from build123d import *

# Parameters (mm, degrees)
SALIENTE_EXTRUIR1_DEPTH = 1400
CROQUIS2_R              = 3
CORTAR_EXTRUIR1_DEPTH   = 1401.160705062
CORTAR_EXTRUIR3_DEPTH   = 1401.160705062
CROQUIS4_W              = 1150
CROQUIS4_H              = 72.748415438
CORTAR_EXTRUIR5_DEPTH   = 254


with BuildPart() as part:
    # Croquis1 → Saliente-Extruir1 (new body)
    with BuildSketch(Plane.XY):
        with BuildLine():
            Line((-14, 15), (14, 15))
            ThreePointArc((14, 15), (14.707106781, 14.707106781), (15, 14))
            Line((15, 14), (15, -14))
            ThreePointArc((15, -14), (14.707106781, -14.707106781), (14, -15))
            Line((14, -15), (-14, -15))
            ThreePointArc((-14, -15), (-14.707106781, -14.707106781), (-15, -14))
            Line((-15, -14), (-15, 14))
            ThreePointArc((-15, 14), (-14.707106781, 14.707106781), (-14, 15))
        make_face()
    extrude(amount=-SALIENTE_EXTRUIR1_DEPTH)

    # Croquis2 → Cortar-Extruir1 (cut, through all)
    with BuildSketch(Plane.XY):
        Circle(CROQUIS2_R)
    extrude(amount=-CORTAR_EXTRUIR1_DEPTH, mode=Mode.SUBTRACT)

    # Croquis3 → Cortar-Extruir3 (cut, through all)
    with BuildSketch(Plane.XY):
        with BuildLine():
            Line((-5.492893219, 4.078679656), (-11.292893219, 9.878679656))
            ThreePointArc((-11.292893219, 9.878679656), (-12.382683432, 10.095452408), (-13, 9.171572875))
            Line((-13, 9.171572875), (-13, 5))
            ThreePointArc((-13, 5), (-14, 4), (-15, 5))
            Line((-15, 5), (-15, -5))
            ThreePointArc((-15, -5), (-14, -4), (-13, -5))
            Line((-13, -5), (-13, -9.171572875))
            ThreePointArc((-13, -9.171572875), (-12.382683432, -10.095452408), (-11.292893219, -9.878679656))
            Line((-11.292893219, -9.878679656), (-5.492893219, -4.078679656))
            ThreePointArc((-5.492893219, -4.078679656), (-5.276120467, -3.754256308), (-5.2, -3.371572875))
            Line((-5.2, -3.371572875), (-5.2, 3.371572875))
            ThreePointArc((-5.2, 3.371572875), (-5.276120467, 3.754256308), (-5.492893219, 4.078679656))
        make_face()
        with BuildLine():
            ThreePointArc((-9.171572875, 13), (-10.095452408, 12.382683432), (-9.878679656, 11.292893219))
            Line((-9.878679656, 11.292893219), (-4.078679656, 5.492893219))
            ThreePointArc((-4.078679656, 5.492893219), (-3.754256308, 5.276120467), (-3.371572875, 5.2))
            Line((-3.371572875, 5.2), (3.371572875, 5.2))
            ThreePointArc((3.371572875, 5.2), (3.754256308, 5.276120467), (4.078679656, 5.492893219))
            Line((4.078679656, 5.492893219), (9.878679656, 11.292893219))
            ThreePointArc((9.878679656, 11.292893219), (10.095452408, 12.382683432), (9.171572875, 13))
            Line((9.171572875, 13), (5, 13))
            ThreePointArc((5, 13), (4, 14), (5, 15))
            Line((5, 15), (-5, 15))
            ThreePointArc((-5, 15), (-4.292893219, 14.707106781), (-4, 14))
            ThreePointArc((-4, 14), (-4.292893219, 13.292893219), (-5, 13))
            Line((-5, 13), (-9.171572875, 13))
        make_face()
        with BuildLine():
            Line((9.878679656, -11.292893219), (4.078679656, -5.492893219))
            ThreePointArc((4.078679656, -5.492893219), (3.754256308, -5.276120467), (3.371572875, -5.2))
            Line((3.371572875, -5.2), (-3.371572875, -5.2))
            ThreePointArc((-3.371572875, -5.2), (-3.754256308, -5.276120467), (-4.078679656, -5.492893219))
            Line((-4.078679656, -5.492893219), (-9.878679656, -11.292893219))
            ThreePointArc((-9.878679656, -11.292893219), (-10.095452408, -12.382683432), (-9.171572875, -13))
            Line((-9.171572875, -13), (-5, -13))
            ThreePointArc((-5, -13), (-4.292893219, -13.292893219), (-4, -14))
            ThreePointArc((-4, -14), (-4.292893219, -14.707106781), (-5, -15))
            Line((-5, -15), (5, -15))
            ThreePointArc((5, -15), (4, -14), (5, -13))
            Line((5, -13), (9.171572875, -13))
            ThreePointArc((9.171572875, -13), (10.095452408, -12.382683432), (9.878679656, -11.292893219))
        make_face()
        with BuildLine():
            ThreePointArc((13, 9.171572875), (12.382683432, 10.095452408), (11.292893219, 9.878679656))
            Line((11.292893219, 9.878679656), (5.492893219, 4.078679656))
            ThreePointArc((5.492893219, 4.078679656), (5.276120467, 3.754256308), (5.2, 3.371572875))
            Line((5.2, 3.371572875), (5.2, -3.371572875))
            ThreePointArc((5.2, -3.371572875), (5.276120467, -3.754256308), (5.492893219, -4.078679656))
            Line((5.492893219, -4.078679656), (11.292893219, -9.878679656))
            ThreePointArc((11.292893219, -9.878679656), (12.382683432, -10.095452408), (13, -9.171572875))
            Line((13, -9.171572875), (13, -5))
            ThreePointArc((13, -5), (14, -4), (15, -5))
            Line((15, -5), (15, 5))
            ThreePointArc((15, 5), (14, 4), (13, 5))
            Line((13, 5), (13, 9.171572875))
        make_face()
    extrude(amount=-CORTAR_EXTRUIR3_DEPTH, mode=Mode.SUBTRACT)

    # Croquis4 → Cortar-Extruir5 (cut)
    with BuildSketch(Plane.ZY.offset(15)):
        with Locations((-825, -21.374207719)):
            Rectangle(CROQUIS4_W, CROQUIS4_H)
    extrude(amount=-CORTAR_EXTRUIR5_DEPTH, mode=Mode.SUBTRACT)


solid = part.part
The listing builds one solid part. Answer for the finished solid, in the listing's coordinates (mm). A direction names the side the tool comes from. Give positions to 0.01 mm unless a question says otherwise; leave off trailing zeros. Write each loop counter-clockwise with the first axis right and the second up, starting at its lowest first coordinate (ties: lowest second). Pieces come first, ordered by that corner, then holes. Notation, with made-up numbers: (-1, -7.5) -> (44, -7.5) arc R28 cw to (44, 13.5) -> close; hole circle Ø11 at (-29, -24). An arc over 180 degrees is marked (long way). Use a Markdown table: item, result.
(1) Flat-ended cylindrical pins translate along their axes: P1, Ø1.5, axis at x = -4, z = -207.5, coming from the -Y side; P2, Ø7.5, axis at y = 0.5, z = -142.5, coming from the -X side; P3, Ø2, axis at x = 1.5, z = -179.5, coming from the +Y side. Find the tip coordinate at first contact, or state that the pin passes through.
Return value:
| item | result |
|---|---|
| P1 | y = -14.97 |
| P2 | x = -14.66 |
| P3 | y = 5.2 |
(2) Determine the mould class of faces 1 (the flat face through (-7, -13, -123)), 2 (the flat face through (-13, -7, -123)), 3 (the flat face through (0, -4, -250)), 4 (the flat face through (5.2, 0, -123)) for opening direction X: released by +X, released by -X, zero draft, split by the parting line, or undercut.
Return value:
| item | result |
|---|---|
| face 1 | undercut |
| face 2 | undercut |
| face 3 | zero draft |
| face 4 | released by +X |
(3) For faces 5 (the flat face through (-15, -10, -123)), 6 (the flat face through (0, -5.2, -123)), 7 (the flat face through (7.019, -8.433, -123.25)), 8 (the flat face through (0, 5.2, -123)), determine the directions among +Z, -Z, +X, -X, +Y, -Y from which every point of the face is accessible in a straight line to the end or side of a thin tool.
Return value:
| item | result |
|---|---|
| face 5 | +Z, -Z, -X, +Y, -Y |
| face 6 | +Z, -Z, -Y |
| face 7 | +Z, -Z |
| face 8 | +Z, -Z, +Y |
(4) Find the intervals of material crossed by probe 1 along Y at (x, z) = (13.75, -158); probe 2 along X at (y, z) = (10, -33.5); probe 3 along Y at (x, z) = (-9, -35.5), in increasing order. Write a range as from..to.
Return value:
| item | result |
|---|---|
| probe 1 | -15..-4.03, 4.03..15 |
| probe 2 | -15..-12.56, -11.44..-8.59, 8.59..11.44, 12.56..15 |
| probe 3 | -15..-13, -10.41..-7.59, 7.59..10.41, 13..15 |
(5) Section A-A, the plane x = 0 is taken. Determine the outline of the cut face in (y, z).
Return value:
| item | result |
|---|---|
| outline | (-5.2, -250) -> (-3, -250) -> (-3, 0) -> (-5.2, 0) -> close; (3, -250) -> (5.2, -250) -> (5.2, 0) -> (3, 0) -> close |
